```python
from build123d import *

# Parameters (mm, degrees)
SKETCH1_R           = 19
BOSS_EXTRUDE1_DEPTH = 27
CUT_EXTRUDE1_START  = -27
SKETCH2_R           = 3
CUT_EXTRUDE1_DEPTH  = 20
BOSS_EXTRUDE2_START = 4
BOSS_EXTRUDE2_DEPTH = 20
FILLET1_R           = 50
FILLET2_R           = 30
FILLET3_R           = 10
FILLET4_R           = 35
FILLET5_R           = 100
FILLET6_R           = 35
FILLET7_R           = 2
FILLET8_R           = 2


with BuildPart() as part:
    # Sketch1 → Boss-Extrude1 (new body)
    with BuildSketch(Plane(origin=(0, 0, 0), x_dir=(0, 0, -1), z_dir=(1, 0, 0))):
        Circle(SKETCH1_R)
    extrude(amount=BOSS_EXTRUDE1_DEPTH)

    # Sketch2 → Cut-Extrude1 (cut)
    with BuildSketch(Plane(origin=(27, 0, 0), x_dir=(0, 0, -1), z_dir=(1, 0, 0)).offset(CUT_EXTRUDE1_START)):
        Circle(SKETCH2_R)
    extrude(amount=CUT_EXTRUDE1_DEPTH, mode=Mode.SUBTRACT)

    # Sketch3 → Boss-Extrude2 (add)
    with BuildSketch(Plane(origin=(0, 0, 0), x_dir=(0, 0, -1), z_dir=(1, 0, 0)).offset(BOSS_EXTRUDE2_START)):
        with BuildLine():
            Line((18.894443628, -2), (30.571757329, -24.105210805))
            Line((30.571757329, -24.105210805), (29.160101789, -64.105210805))
            Line((29.160101789, -64.105210805), (70.877132442, -80.977950757))
            Line((70.877132442, -80.977950757), (71.761340874, -80.510858209))
            Line((71.761340874, -80.510858209), (113.01650789, -105.296253694))
            ThreePointArc((113.01650789, -105.296253694), (139.2516778, -125.255736415), (160.530160786, -150.432933488))
            Line((160.530160786, -150.432933488), (156.644610862, -153.579757568))
            Line((156.644610862, -153.579757568), (101.784019397, -120.620456846))
            Line((101.784019397, -120.620456846), (37.657121196, -105.296253694))
            Line((37.657121196, -105.296253694), (9.210363464, -86.510744513))
            Line((9.210363464, -86.510744513), (-0.574058656, -56.0433015))
            Line((-0.574058656, -56.0433015), (0.308226057, -31.0433015))
            Line((0.308226057, -31.0433015), (-6.698162164, -17.780175017))
            Line((-6.698162164, -17.780175017), (18.894443628, -2))
        make_face()
    extrude(amount=BOSS_EXTRUDE2_DEPTH)

    # Fillet1
    fillet1_edges = [part.edges().sort_by_distance(p)[0] for p in [
        (14, -24.105210805, -30.571757329),
    ]]
    fillet(fillet1_edges, radius=FILLET1_R)

    # Fillet2
    fillet2_edges = [part.edges().sort_by_distance(p)[0] for p in [
        (14, -31.0433015, -0.308226057),
    ]]
    fillet(fillet2_edges, radius=FILLET2_R)

    # Fillet3
    fillet3_edges = [part.edges().sort_by_distance(p)[0] for p in [
        (14, -56.0433015, 0.574058656),
    ]]
    fillet(fillet3_edges, radius=FILLET3_R)

    # Fillet4
    fillet4_edges = [part.edges().sort_by_distance(p)[0] for p in [
        (14, -86.510744513, -9.210363464),
    ]]
    fillet(fillet4_edges, radius=FILLET4_R)

    # Fillet5
    fillet5_edges = [part.edges().sort_by_distance(p)[0] for p in [
        (14, -105.296253694, -37.657121196),
        (14, -120.620456846, -101.784019397),
    ]]
    fillet(fillet5_edges, radius=FILLET5_R)

    # Fillet6
    fillet6_edges = [part.edges().sort_by_distance(p)[0] for p in [
        (14, -64.105210805, -29.160101789),
    ]]
    fillet(fillet6_edges, radius=FILLET6_R)

    # Fillet7
    fillet7_edges = [part.edges().sort_by_distance(p)[0] for p in [
        (14, -80.977950757, -70.877132442),
    ]]
    fillet(fillet7_edges, radius=FILLET7_R)

    # Fillet8
    fillet8_edges = [part.edges().sort_by_distance(p)[0] for p in [
        (4, -20.874395385, 5.063607207),
        (14, -153.579757568, -156.644610862),
        (4, -80.527255596, -71.730300543),
        (24, -20.874395385, 5.063607207),
        (24, -80.527255596, -71.730300543),
        (4, -7.157033947, -21.61870189),
        (24, -7.157033947, -21.61870189),
        (4, -24.495759346, -28.868208254),
        (24, -24.495759346, -28.868208254),
        (4, -46.668154937, 0.243196716),
        (24, -46.668154937, 0.243196716),
        (4, -31.277630624, 0.713903389),
        (24, -31.277630624, 0.713903389),
        (4, -66.24854061, -2.70328783),
        (24, -66.24854061, -2.70328783),
        (4, -56.022494361, 0.423944925),
        (24, -56.022494361, 0.423944925),
        (4, -94.437046571, -21.213104097),
        (24, -94.437046571, -21.213104097),
        (4, -85.240499997, -10.884930764),
        (24, -85.240499997, -10.884930764),
        (4, -141.076434231, -135.832891606),
        (24, -141.076434231, -135.832891606),
        (4, -113.212895767, -70.785741018),
        (24, -113.212895767, -70.785741018),
        (4, -103.880894632, -38.270767893),
        (24, -103.880894632, -38.270767893),
        (4, -121.717757742, -101.335811711),
        (24, -121.717757742, -101.335811711),
        (4, -38.522680641, -30.0629448),
        (24, -38.522680641, -30.0629448),
        (4, -59.899123869, -35.642159411),
        (24, -59.899123869, -35.642159411),
        (4, -76.961765139, -60.947308417),
        (24, -76.961765139, -60.947308417),
        (4, -80.772653132, -70.866688464),
        (24, -80.772653132, -70.866688464),
    ]]
    fillet(fillet8_edges, radius=FILLET8_R)


solid = part.part
```
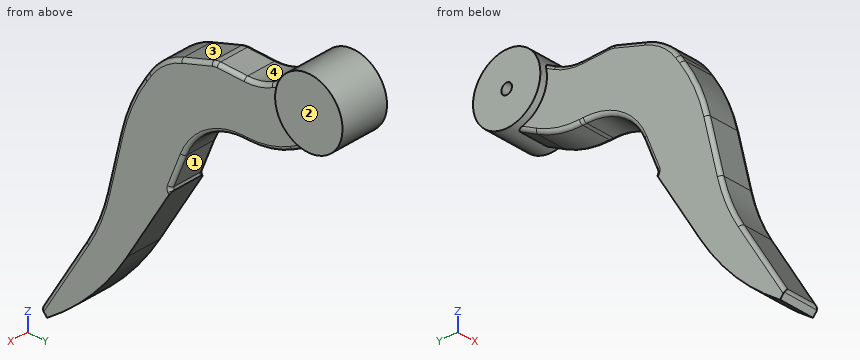
Source: CAD feature listing. Evaluate the final solid. Frame: model axes, mm. Face numbers are marked on the shaded views. Give positions to 0.01 mm unless a question says otherwise; leave off trailing zeros. Write each loop counter-clockwise with the first axis right and the second up, starting at its lowest first coordinate (ties: lowest second). Pieces come first, ordered by that corner, then holes.
1. Pull-direction query (Y, two-part tool) for the marked faces 1, 2, 3 and 4; classes: +Y half, -Y half, draft (parallel to the pull), parting line (faces both ways), or undercut.
2. First-contact query: pin 1 (5 mm diameter, centred on x = 19.5, y = -40.5, fed in from -Z); pin 2 (1.5 mm diameter, centred on x = 3.5, z = -108, fed in from -Y); pin 3 (4 mm diameter, centred on y = -43.5, z = -16, fed in from -X). Flat tips, straight axial feed; report the tip coordinate or a pass-through.
3. Section query A-A (x = 8.25). Return the cut outline in (y, z).
4. Material intervals for line 1 along X through (y, z) = (-21.5, -8); line 2 along Z through (x, y) = (19.75, -135.5); line 3 along Z through (x, y) = (13.5, -12.5), sorted ascending.
Output values:
1. face 1: +Y half
1. face 2: draft
1. face 3: -Y half
1. face 4: undercut
2. pin 1: stops at z = -30.08
2. pin 2: stops at y = -123.62
2. pin 3: stops at x = 4
3. outline: (-152.86, -155.44) arc R2 ccw to (-152.7, -157.73) - (-150.43, -160.53) arc R150.99 ccw to (-105.3, -113.02) - (-80.51, -71.76) - (-80.54, -71.7) arc R2 cw to (-80.63, -70.02) - (-73.29, -51.88) arc R35 cw to (-39.61, -30.02) - (-37.43, -30.1) arc R50 ccw to (-12.31, -24.34) - (-2, -18.89) arc R19 ccw (long way) to (-17.78, 6.7) - (-23.97, 3.43) arc R30 cw to (-39.04, -0.03) - (-54.3, 0.51) arc R10 ccw to (-57.71, 0.04) - (-74.79, -5.45) arc R35 ccw to (-93.29, -19.48) - (-95.58, -22.94) arc R100 ccw to (-109.39, -54.81) - (-117.03, -86.76) arc R100 cw to (-128.57, -115.02) - close; hole circle Ø6 at (0, 0)
4. line 1: x = 4 to 24
4. line 2: z = -149.07 to -126.55
4. line 3: z = -24.44 to 14.31
